Input: part model. Units: mm. Frame: model coordinates. A direction names the side the tool comes from. Coordinates: 2 decimals unless noted, no trailing zeros. Order: outer loops, then holes, each group sorted by start corner. A loop starts at its lowest first (then second) coordinate and runs counter-clockwise, first axis right, second up. Notation, with made-up numbers: (-28, 75.25) -> (-7, 75.25) arc R21 cw to (-7, 93.25) -> close; hole circle Ø8 at (-36, -17.5). An arc over 180 degrees is marked (long way). One line per question, with ' | ' between items.
```python
from build123d import *

# Parameters (mm, degrees)
F0_W     = 88.9
F0_H     = 127
F1_DEPTH = 3.175
F2_W     = 88.9
F2_H     = 17.9578
F3_DEPTH = 17.9578
F4_SIZE  = 17.95779
F5_R     = 25.4
F6_DEPTH = 3.175
F7_W     = 88.9
F7_H     = 12.7
F8_DEPTH = 12.7
F9_SIZE2 = 12.69999
F9_SIZE  = 2.53999


# Not quite as in the source:
# - a fillet or chamfer is up to 0.001 mm smaller than in the source, because OpenCascade refuses the exact size


with BuildPart() as f1:
    # F0 (on Top) → F1 (new body)
    with BuildSketch(Plane.XY):
        Rectangle(F0_W, F0_H)
    extrude(amount=F1_DEPTH)

    # F2 (on face) → F3 (join)
    with BuildSketch(Plane(origin=(0, 0, 0), x_dir=(1, 0, 0), z_dir=(0, 0, -1))):
        with Locations((0, -54.5211)):
            Rectangle(F2_W, F2_H)
    extrude(amount=F3_DEPTH)

    # F4 (size 17.9578 in the source; OpenCascade refuses exactly that, so slightly less here)
    f4_edges = [f1.edges().sort_by_distance(p)[0] for p in [
        (0, 63.5, -17.9578),
    ]]
    chamfer(f4_edges, length=F4_SIZE)

    # F5 (on face) → F6 (cut)
    with BuildSketch(Plane.XY.offset(3.175)):
        Circle(F5_R)
    extrude(amount=-F6_DEPTH, mode=Mode.SUBTRACT)

    # F7 (on face) → F8 (join)
    with BuildSketch(Plane.XY.offset(3.175)):
        with Locations((0, -57.15)):
            Rectangle(F7_W, F7_H)
    extrude(amount=F8_DEPTH)

    # F9 (size 2.54 and 12.7 in the source; OpenCascade refuses exactly that, so slightly less here)
    f9_edges = [f1.edges().sort_by_distance(p)[0] for p in [
        (0, -50.8, 15.875),
    ]]
    f9_side = f1.faces().sort_by_distance((0, -57.15, 15.875))[0]
    chamfer(f9_edges, length=F9_SIZE, length2=F9_SIZE2, reference=f9_side)


solid = f1.part
```
1. Ray query, line 1 (Y direction, x = 0, z = 2); line 2 (Z direction, x = -31, y = -3.5) (3 decimals); line 3 (Z direction, x = -3, y = 56) (3 decimals). Return the intervals inside material, ascending. Write a range as [from, to].
Recorded:
line 1: y = [-63.5, -25.4], [25.4, 63.5] | line 2: z = [0, 3.175] | line 3: z = [-7.5, 3.175]
2. Cut plane B-B, the plane y = 0. Return loops of the section in (x, z) (3 decimals).
Recorded:
outline: (-44.45, 0) -> (-25.4, 0) -> (-25.4, 3.175) -> (-44.45, 3.175) -> close; (25.4, 0) -> (44.45, 0) -> (44.45, 3.175) -> (25.4, 3.175) -> close
3. Access query for faces 5 (the face through (-1, 45.542, -9)), 6 (the face through (-1, -63.5, 8)), 7 (the face through (19, 20, 3.175)). Directions: +Z, -Z, +X, -X, +Y, -Y. A direction counts if a zero-diameter tool reaches every point of the face in a straight line with its end or side. Return the directions, or none.
Recorded:
face 5: -Z, +X, -X, -Y | face 6: +Z, -Z, +X, -X, -Y | face 7: +Z, +X, -X, +Y
4. Mould query, pull axis X, two halves, no side actions, for faces 1 (the face through (44.45, 0, 3)), 2 (the face through (-44.45, 0, 3)), 3 (the face through (-0.6, 54.4, -9.1)), 4 (the face through (-5.506, -24.796, 1.61)). Classes: released by +X, released by -X, zero draft, split by the parting line, or undercut.
Recorded:
face 1: released by +X | face 2: released by -X | face 3: zero draft | face 4: undercut
5. Pin query (flat end, axial travel): pin 1 Ø1 at (x, z) = (18, -2.5) entering from -Y; pin 2 Ø10 at (y, z) = (0, -0.5) entering from +X; pin 3 Ø12 at (x, z) = (10, -9.5) entering from +Y; pin 4 Ø1 at (x, y) = (-15, -42) entering from +Z (3 decimals). Return the tip coordinate at first contact, or that it passes through.
Recorded:
pin 1: stops at y = 45.54 | pin 2: stops at x = 44.45 | pin 3: stops at y = 60 | pin 4: stops at z = 3.175
